```python
from build123d import *

# Parameters (mm, degrees)
SKETCH_1_R      = 11
SKETCH_1_R_2    = 9
EXTRUDE_1_DEPTH = 248
EXTRUDE_START   = 12
SKETCH_2_R      = 11
EXTRUDE_2_DEPTH = 12
SKETCH_4_R      = 4
EXTRUDE_4_DEPTH = 2.5
SKETCH_5_R      = 11
SKETCH_5_R_2    = 6
EXTRUDE_5_DEPTH = 5


with BuildPart() as part:
    # 草圖1 → 填料-伸長1 (new body)
    with BuildSketch(Plane(origin=(0, 0, 0), x_dir=(1, 0, 0), z_dir=(0, 1, 0))):
        with Locations(Location((0, 0, 0), (0, 0, 270))):
            Circle(SKETCH_1_R)
        with Locations(Location((0, 0, 0), (0, 0, 270))):
            Circle(SKETCH_1_R_2, mode=Mode.SUBTRACT)
    extrude(amount=EXTRUDE_1_DEPTH)

    # 草圖2 → 填料-伸長2 (add)
    with BuildSketch(Plane.XZ.offset(EXTRUDE_START)):
        with Locations(Location((0, 0, 0), (0, 0, 270))):
            Circle(SKETCH_2_R)
    extrude(amount=-EXTRUDE_2_DEPTH)

    # 草圖4 → 填料-伸長4 (add, symmetric)
    with BuildSketch(Plane(origin=(0, 0, 0), x_dir=(0, 0, -1), z_dir=(1, 0, 0))):
        with BuildLine():
            Line((-7, -12), (-7, -25))
            ThreePointArc((-7, -25), (0, -32), (7, -25))
            Line((7, -25), (7, -12))
            Line((7, -12), (-7, -12))
        make_face()
        with Locations((0, -25)):
            Circle(SKETCH_4_R, mode=Mode.SUBTRACT)
    extrude(amount=EXTRUDE_4_DEPTH, both=True)

    # 草圖5 → 填料-伸長5 (add)
    with BuildSketch(Plane(origin=(0, 248, 0), x_dir=(1, 0, 0), z_dir=(0, 1, 0))):
        with Locations(Location((0, 0, 0), (0, 0, 90))):
            Circle(SKETCH_5_R)
        with Locations(Location((0, 0, 0), (0, 0, 270))):
            Circle(SKETCH_5_R_2, mode=Mode.SUBTRACT)
    extrude(amount=EXTRUDE_5_DEPTH)


solid = part.part
```
Work out the finished part from the listing and answer in its coordinate system (mm). A direction names the side the tool comes from. Give positions to 0.01 mm unless a question says otherwise; leave off trailing zeros. Loops run counter-clockwise (first coordinate to the right, second up) from the corner with the lowest first, then second, coordinate; pieces in that order, holes last. Notation, with made-up numbers: (-32, 55.5) - (24, 55.5) arc R11 cw to (24, 74.5) - close; hole circle Ø6 at (88.25, 20). An arc over 180 degrees is marked (long way). Use CSV: the item, a comma, the result in double quotes. Start each with the question number.
(1) Find the intervals of material crossed by L1, parallel to Y at x = -5.5, z = -3.5; L2, parallel to X at y = 86, z = 0; L3, parallel to Y at x = -0.8, z = 0, in increasing order.
(2) Find section C-C, the plane y = 190.5. Determine the outline of the cut face in (x, z).
(3) Find section B-B, the plane x = 0. Determine the outline of the cut face in (y, z), plus the area to 3 significant figures.
(4) A tool of negligible diameter and unlimited length cuts with its end or side. For faces 1 (the face through (0, -19, -7)), 2 (the face through (1.802, 250.465, 5.723)), 3 (the face through (0, -18, 7)), 4 (the face through (2.703, 122.264, 8.584)), from which of +Z, -Z, +X, -X, +Y, -Y can it reach the whole face along a straight path? Write none if from no direction.
(5) Find section A-A, the plane z = 0. Determine the outline of the cut face in (x, y), plus the area to 3 significant figures.
(6) Determine the mould class of faces 5 (the face through (6, 248, -2)), 6 (the face through (0, -32, 0)), 7 (the face through (2.5, -20, 0)) for opening direction Y: released by +Y, released by -Y, zero draft, split by the parting line, or undercut.
(7) Each of these flat-tipped pins is pushed along its axis until it touches: pin 1 (13 mm diameter, centred on y = -25, z = 0, fed in from -X); pin 2 (1.5 mm diameter, centred on y = 63.5, z = 6, fed in from +X); pin 3 (1 mm diameter, centred on y = 108.5, z = 4.5, fed in from +X). Where does it stop, or does it pass through?
Results found:
1,L1,"-12 to 0, 248 to 253"
1,L2,"-11 to -9, 9 to 11"
1,L3,"-32 to -29, -21 to 0"
2,outline,"circle Ø22 at (0, 0); hole circle Ø18 at (0, 0)"
3,outline,"(-25, -7) - (-12, -7) - (-12, -11) - (253, -11) - (253, -6) - (248, -6) - (248, -9) - (0, -9) - (0, 9) - (248, 9) - (248, 6) - (253, 6) - (253, 11) - (-12, 11) - (-12, 7) - (-25, 7) arc R7 ccw to start; hole circle Ø8 at (-25, 0)"
3,area,"1,510 mm^2"
4,face 1,"-Z, +X, -X, -Y"
4,face 2,"+Y"
4,face 3,"+Z, +X, -X, -Y"
4,face 4,"none"
5,outline,"(-11, -12) - (-2.5, -12) - (-2.5, -21) - (2.5, -21) - (2.5, -12) - (11, -12) - (11, 253) - (6, 253) - (6, 248) - (9, 248) - (9, 0) - (-9, 0) - (-9, 248) - (-6, 248) - (-6, 253) - (-11, 253) - close; (-2.5, -32) - (2.5, -32) - (2.5, -29) - (-2.5, -29) - close"
5,area,"1,370 mm^2"
6,face 5,"undercut"
6,face 6,"released by -Y"
6,face 7,"zero draft"
7,pin 1,"x = -2.5"
7,pin 2,"x = 9.67"
7,pin 3,"x = 10.25"
